Drawing for the job (mm, zero at the part's lowest x, y, z). Round coordinates to 2 decimals unless told otherwise and drop trailing zeros. Write each loop counter-clockwise with the first axis right and the second up, starting at its lowest first coordinate (ties: lowest second). Pieces come first, ordered by that corner, then holes.
Item 1: Band-saw the part on C-C, the plane x = 97. Write the cut outline in (y, z).
Item 2: Wall check: probe 1 along Y at (x, z) = (142, 11); probe 2 along X at (y, z) = (106.5, 9.75); probe 3 along Z at (x, y) = (160, 92.5). Give the ranges that are in metal, low to high.
Item 3: Band-saw the part on A-A, the plane x = 63. Write the cut outline in (y, z).
Item 4: Band-saw the part on B-B, the plane y = 121.5. Write the cut outline in (x, z).
Item 5: Drop flat-ended pins along their axis: pin 1 Ø4 at (x, z) = (19.5, 10) entering from +Y; pin 2 Ø1 at (y, z) = (69.5, 10) entering from +X; pin 3 Ø0.6 at (y, z) = (60.5, 9.5) entering from +X. Give the stop position or say it passes through.
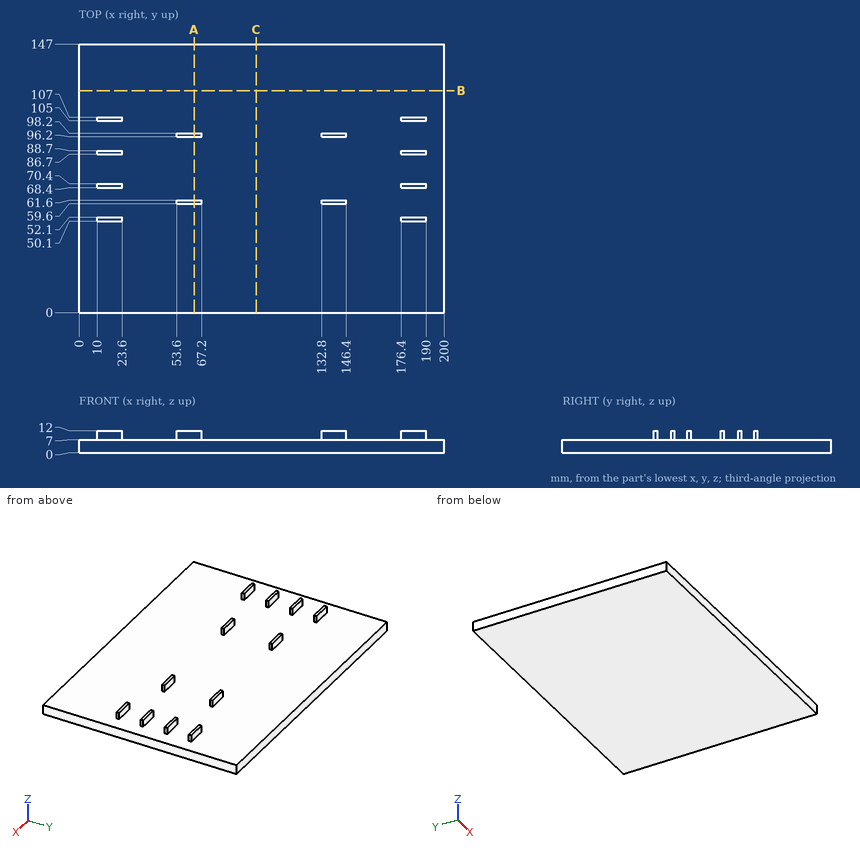
Results:
1. outline: (0, 0) - (147, 0) - (147, 7) - (0, 7) - close
2. probe 1: y = 59.6 to 61.6, 96.2 to 98.2
2. probe 2: x = 10 to 23.6, 176.4 to 190
2. probe 3: z = 0 to 7
3. outline: (0, 0) - (147, 0) - (147, 7) - (98.2, 7) - (98.2, 12) - (96.2, 12) - (96.2, 7) - (61.6, 7) - (61.6, 12) - (59.6, 12) - (59.6, 7) - (0, 7) - close
4. outline: (0, 0) - (200, 0) - (200, 7) - (0, 7) - close
5. pin 1: stops at y = 107
5. pin 2: stops at x = 190
5. pin 3: stops at x = 146.4
